from build123d import *

# Parameters (mm, degrees)
BOSS_EXTRUDE2_DEPTH                = 7
SKETCH3_W                          = 27
SKETCH3_H                          = 3
CUT_EXTRUDE2_DEPTH                 = 10
F_3_5_START                        = -16.5
F_3_5_3_5_DIAMETER_HOLE1_OUTLINE_R = 1.75
F_3_5_3_5_DIAMETER_HOLE1_DEPTH     = 33
BOSS_EXTRUDE4_DEPTH                = 1


# Read off the part's stored shape, not the designer's step: Ø3.5 (3.5) Diameter Hole1
with BuildPart() as part:
    # Sketch1 → Boss-Extrude2 (new body)
    # profile 1 of 5: a face of its own
    with BuildSketch(Plane(origin=(0, 0, 0), x_dir=(1, 0, 0), z_dir=(0, 1, 0))):
        with BuildLine():
            ThreePointArc((87.751176684, -3), (0, 94.211501571), (-87.751176684, -3))
            Line((-87.751176684, -3), (87.751176684, -3))
        make_face()
        with BuildLine():
            Line((-16.5, 0), (-85, 0))
            ThreePointArc((-85, 0), (-80.982173458, 32.512027121), (-64.995192411, 61.105580148))
            ThreePointArc((-64.995192411, 61.105580148), (-64.013019257, 62.243518432), (-63.01092574, 63.363954164))
            ThreePointArc((-63.01092574, 63.363954164), (-35.129795909, 83.633095001), (-1.5, 91.198298105))
            ThreePointArc((-1.5, 91.198298105), (0, 91.211501571), (1.5, 91.198298105))
            ThreePointArc((1.5, 91.198298105), (35.129795909, 83.633095001), (63.01092574, 63.363954164))
            ThreePointArc((63.01092574, 63.363954164), (64.013019257, 62.243518432), (64.995192411, 61.105580148))
            ThreePointArc((64.995192411, 61.105580148), (80.982173458, 32.512027121), (85, 0))
            Line((85, 0), (16.5, 0))
            Line((16.5, 0), (13.5, 0))
            Line((13.5, 0), (-13.5, 0))
            Line((-13.5, 0), (-16.5, 0))
        make_face(mode=Mode.SUBTRACT)
    # profile 2 of 5: a face of its own
    with BuildSketch(Plane(origin=(0, 0, 0), x_dir=(1, 0, 0), z_dir=(0, 1, 0))):
        with BuildLine():
            Line((16.5, 14.73170808), (16.5, 12.610387736))
            Line((16.5, 12.610387736), (64.995192411, 61.105580148))
            ThreePointArc((64.995192411, 61.105580148), (64.013019257, 62.243518432), (63.01092574, 63.363954164))
            Line((63.01092574, 63.363954164), (15.155331601, 15.508360024))
            Line((15.155331601, 15.508360024), (16.5, 14.73170808))
        make_face()
    # profile 3 of 5: a face of its own
    with BuildSketch(Plane(origin=(0, 0, 0), x_dir=(1, 0, 0), z_dir=(0, 1, 0))):
        with BuildLine():
            ThreePointArc((1.5, 91.198298105), (0, 91.211501571), (-1.5, 91.198298105))
            Line((-1.5, 91.198298105), (-1.5, 23.395389902))
            Line((-1.5, 23.395389902), (0, 24.261758084))
            Line((0, 24.261758084), (1.5, 23.395389902))
            Line((1.5, 23.395389902), (1.5, 91.198298105))
        make_face()
    # profile 4 of 5: a face of its own
    with BuildSketch(Plane(origin=(0, 0, 0), x_dir=(1, 0, 0), z_dir=(0, 1, 0))):
        with BuildLine():
            ThreePointArc((-63.01092574, 63.363954164), (-64.013019257, 62.243518432), (-64.995192411, 61.105580148))
            Line((-64.995192411, 61.105580148), (-16.5, 12.610387736))
            Line((-16.5, 12.610387736), (-16.5, 14.73170808))
            Line((-16.5, 14.73170808), (-15.155331601, 15.508360024))
            Line((-15.155331601, 15.508360024), (-63.01092574, 63.363954164))
        make_face()
    # profile 5 of 5: a face of its own
    with BuildSketch(Plane(origin=(0, 0, 0), x_dir=(1, 0, 0), z_dir=(0, 1, 0))):
        Polygon((-16.5, 12.610387736), (-16.5, 0), (-13.5, 0), (-13.5, 13), (0, 20.79731364), (13.5, 13), (13.5, 0), (16.5, 0), (16.5, 12.610387736), (16.5, 14.73170808), (15.155331601, 15.508360024), (1.5, 23.395389902), (0, 24.261758084), (-1.5, 23.395389902), (-15.155331601, 15.508360024), (-16.5, 14.73170808), align=None)
    extrude(amount=BOSS_EXTRUDE2_DEPTH)

    # Sketch3 → Cut-Extrude2 (cut)
    with BuildSketch(Plane(origin=(0, 7, 0), x_dir=(1, 0, 0), z_dir=(0, 1, 0))):
        with Locations((0, -1.5)):
            Rectangle(SKETCH3_W, SKETCH3_H)
    extrude(amount=-CUT_EXTRUDE2_DEPTH, mode=Mode.SUBTRACT)

    # Ø3.5 (3.5) Diameter Hole1 outline → Ø3.5 (3.5) Diameter Hole1 (cut)
    with BuildSketch(Plane.YZ.offset(F_3_5_START)):
        with Locations((3, -5.010387736)):
            Circle(F_3_5_3_5_DIAMETER_HOLE1_OUTLINE_R)
    extrude(amount=F_3_5_3_5_DIAMETER_HOLE1_DEPTH, mode=Mode.SUBTRACT)

    # Sketch6 → Boss-Extrude4 (add)
    with BuildSketch(Plane(origin=(0, 7, 0), x_dir=(1, 0, 0), z_dir=(0, 1, 0))):
        Polygon((11.5, 11.845527947), (11.5, -3), (13.5, -3), (13.5, 13), (0, 20.79731364), (-13.5, 13), (-13.5, -3), (-11.5, -3), (-11.5, 11.845527947), (0, 18.48768401), align=None)
    extrude(amount=-BOSS_EXTRUDE4_DEPTH)


solid = part.part
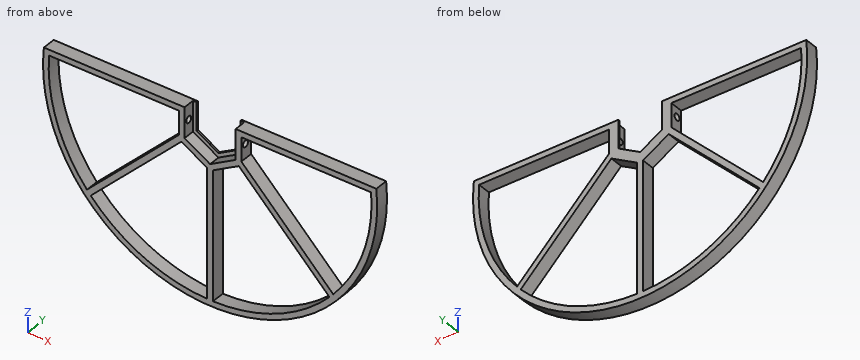
Geometry: final body of the model. Coordinates: model frame, mm. Give positions to 0.01 mm unless a question says otherwise; leave off trailing zeros. Order: outer loops, then holes, each group sorted by start corner. A loop starts at its lowest first (then second) coordinate and runs counter-clockwise, first axis right, second up. Notation, with made-up numbers: (34.25, -21.75) -> (86.25, -21.75) arc R29 cw to (86.25, 14.25) -> close; hole circle Ø10 at (41.25, 41.25). An arc over 180 degrees is marked (long way). Answer as a JSON object with one key per item and string values.
Q1. Section D-D (z = -47). Output: boundary loops of the cut face in (x, y).
Entries:
{"outline": "(-78.1, 0) -> (-74.7, 0) -> (-74.7, 7) -> (-78.1, 7) -> close; (-50.89, 0) -> (-46.65, 0) -> (-46.65, 7) -> (-50.89, 7) -> close; (-1.5, 0) -> (1.5, 0) -> (1.5, 7) -> (-1.5, 7) -> close; (46.65, 0) -> (50.89, 0) -> (50.89, 7) -> (46.65, 7) -> close; (74.7, 0) -> (78.1, 0) -> (78.1, 7) -> (74.7, 7) -> close"}
Q2. Section A-A (y = 3). State how many separate pieces and enclosed holes the cut face has, plus the area to 3 significant figures.
Entries:
{"separate pieces": "1", "enclosed holes": "2", "area": "2,070 mm^2"}
Q3. Material intervals for probe 1 along X at (y, z) = (1, -5.5); probe 2 along Z at (x, y) = (-15.7, 3); probe 3 along Z at (x, y) = (23.5, 5), sorted ascending.
Entries:
{"probe 1": "x = -88.21 to -85.21, -16.5 to -13.5, 13.5 to 16.5, 85.21 to 88.21", "probe 2": "z = -92.8 to -89.75, -16.05 to -6.76, -3.26 to 3", "probe 3": "z = -91.02 to -87.91, -23.85 to -19.61, 0 to 3"}
Q4. Section B-B (x = -72). Output: boundary loops of the cut face in (y, z).
Entries:
{"outline": "(0, -56.96) -> (7, -56.96) -> (7, -51.57) -> (0, -51.57) -> close; (0, 0) -> (7, 0) -> (7, 3) -> (0, 3) -> close"}
Q5. Section C-C (z = -72). Output: boundary loops of the cut face in (x, y), plus the area to 3 significant figures.
Entries:
{"outline": "(-58.53, 0) -> (-53.9, 0) -> (-53.9, 7) -> (-58.53, 7) -> close; (-1.5, 0) -> (1.5, 0) -> (1.5, 7) -> (-1.5, 7) -> close; (53.9, 0) -> (58.53, 0) -> (58.53, 7) -> (53.9, 7) -> close", "area": "85.8 mm^2"}
Q6. First-contact query: pin 1 (2 mm diameter, centred on y = 4.5, z = -6.5, fed in from +X); pin 2 (1.5 mm diameter, centred on x = -39.5, y = 5, fed in from -Z); pin 3 (2 mm diameter, centred on x = -39, y = 2, fed in from -Z). Flat tips, straight axial feed; report the tip coordinate or a pass-through.
Entries:
{"pin 1": "stops at x = 88.21", "pin 2": "stops at z = -85.24", "pin 3": "stops at z = -85.61"}
